Can you work these out from the model? Positions are in its coordinate system, mm. Round coordinates to 2 decimals unless told otherwise and drop trailing zeros. Order: outer loops, then holes, each group sorted by start corner. A loop starts at its lowest first (then second) coordinate and runs counter-clockwise, first axis right, second up.
Autodesk Fusion 360 part; units mm, degrees
sketch "Sketch1" plane through (0, 0, 0) normal (0, 0, 1) x (1, 0, 0)
  line L0 (0, 0) -> (180, 0)
  line L1 (180, 0) -> (180, -12)
  line L2 (180, -12) -> (0, -12)
  line L3 (0, -12) -> (0, 0)
  dimension "d16" = 180
  dimension "d17" = 12
extrude "Extrude1" add sketch "Sketch1" along normal blind 10
sketch "Sketch6" plane through (0, 0, 10) normal (0, 0, 1) x (-1, 0, 0)
  line L0 (0, 12) -> (-180, 12)
  line L1 (-180, 12) -> (-180, 0)
  line L2 (-180, 0) -> (0, 0)
  line L3 (0, 0) -> (0, 12)
  circle A0 centre (-4.7, 6) radius 1.5
  circle A1 centre (-4.7, 6) radius 2.7
  circle A2 centre (-175.3, 6) radius 1.5
  circle A3 centre (-175.3, 6) radius 2.7
  line L4 (0, 12) -> (0, 0)
  line L5 (0, 0) -> (-180, 0)
  line L6 (-180, 0) -> (-180, 12)
  dimension "d65" = 3
  dimension "d66" = 1.2
  dimension "d67" = 3
  dimension "d68" = 1.2
  dimension "d69" = 4.7
  dimension "d70" = 6
  dimension "d71" = 4.7
  dimension "d72" = 6
extrude "Extrude9" cut sketch "Sketch6" against normal blind 100 contours A2
extrude "Extrude10" cut sketch "Sketch6" against normal blind 4 contours A3
extrude "Extrude11" cut sketch "Sketch6" against normal blind 100 contours A0
extrude "Extrude12" cut sketch "Sketch6" against normal blind 4 contours A1
equation "length = 180 mm"
equation "height = 10 mm"
equation "width = 12 mm"
equation "d16 = length"
equation "d17 = width"
equation "d18 = height"
equation "extra = 100 mm"
equation "bearing_outer_radius = 2.7 mm"
equation "bearing_width = 4 mm"
equation "bearing_big_distance = 2 mm + bearing_outer_radius"
equation "bearing_small_distance = width / 2"
equation "bearing_inner_radius = 1.5 mm"
equation "d65 = bearing_inner_radius * 2"
equation "d66 = bearing_outer_radius - bearing_inner_radius"
equation "d67 = bearing_inner_radius * 2"
equation "d68 = bearing_outer_radius - bearing_inner_radius"
equation "d69 = bearing_big_distance"
equation "d70 = bearing_small_distance"
equation "d71 = bearing_big_distance"
equation "d72 = bearing_small_distance"
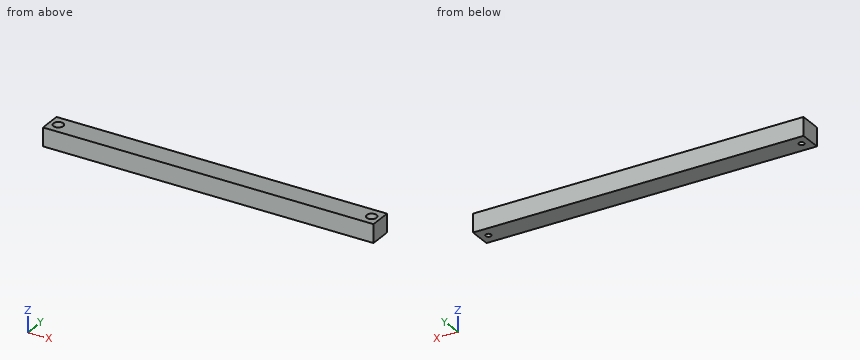
(1) Please list where these lines run through material, in increasing order: probe 1 along X at (y, z) = (-6, 1.4); probe 2 along X at (y, z) = (-6, 8.05); probe 3 along Y at (x, z) = (4.7, 3.4).
(2) I'm going to push a flat-ended pin straight in: pin 1 Ø1.8 at (x, y) = (175.3, -6) entering from -Z. Where does the tip first touch, or does it pass through?
(3) I want a section at A-A, the plane y = -6. List the corners of the cut face in (x, z) for me.
(4) I want a section at B-B, the plane x = 4.7. List the corners of the cut face in (y, z) for me, plus the area to 3 significant figures.
(5) I want a section at C-C, the plane z = 8.5. List the corners of the cut face in (x, y) for me, plus the area to 3 significant figures.
Ans:
1. probe 1: x = 0 to 3.2, 6.2 to 173.8, 176.8 to 180
1. probe 2: x = 0 to 2, 7.4 to 172.6, 178 to 180
1. probe 3: y = -12 to -7.5, -4.5 to 0
2. pin 1: passes through
3. outline: (0, 0) - (3.2, 0) - (3.2, 6) - (2, 6) - (2, 10) - (0, 10) - close; (6.2, 0) - (173.8, 0) - (173.8, 6) - (172.6, 6) - (172.6, 10) - (7.4, 10) - (7.4, 6) - (6.2, 6) - close; (176.8, 0) - (180, 0) - (180, 10) - (178, 10) - (178, 6) - (176.8, 6) - close
4. outline: (-12, 0) - (-7.5, 0) - (-7.5, 6) - (-8.7, 6) - (-8.7, 10) - (-12, 10) - close; (-4.5, 0) - (0, 0) - (0, 10) - (-3.3, 10) - (-3.3, 6) - (-4.5, 6) - close
4. area: 80.4 mm2
5. outline: (0, -12) - (180, -12) - (180, 0) - (0, 0) - close; hole circle Ø5.4 at (4.7, -6); hole circle Ø5.4 at (175.3, -6)
5. area: 2,110 mm2
